```python
from build123d import *

# Parameters (mm, degrees)
BOSS_EXTRUDE1_DEPTH            = 2.54
F_3_16_0_1875_DIAMETER_HOLE1_D = 4.7625
CHAMFER1_SIZE                  = 2.54
CHAMFER2_SIZE                  = 0.2


with BuildPart() as part:
    # Sketch1 → Boss-Extrude1 (new body)
    with BuildSketch(Plane(origin=(0, 0, 0), x_dir=(1, 0, 0), z_dir=(0, 1, 0))):
        Polygon((0, 0), (-25.4, 0), (-25.4, -25.4), (50.8, -25.4), (50.8, 0), (25.4, 0), (25.4, 50.8), (0, 50.8), align=None)
    extrude(amount=BOSS_EXTRUDE1_DEPTH)

    # 3/16 (0.1875) Diameter Hole1 (through all)
    with Locations(Plane(origin=(0, 2.54, 0), x_dir=(1, 0, 0), z_dir=(0, 1, 0))):
        with Locations((12.7, 38.1), (12.7, 12.7), (12.7, -12.7), (38.1, -12.7), (-12.7, -12.7)):
            Hole(F_3_16_0_1875_DIAMETER_HOLE1_D / 2)

    # Chamfer1
    chamfer1_edges = [part.edges().sort_by_distance(p)[0] for p in [
        (0, 1.27, -50.8),
        (25.4, 1.27, -50.8),
        (25.4, 1.27, 0),
        (50.8, 1.27, 0),
        (50.8, 1.27, 25.4),
        (-25.4, 1.27, 25.4),
        (-25.4, 1.27, 0),
        (0, 1.27, 0),
    ]]
    chamfer(chamfer1_edges, length=CHAMFER1_SIZE)

    # Chamfer2
    chamfer2_edges = [part.edges().sort_by_distance(p)[0] for p in [
        (-10.31875, 2.54, 12.7),
        (-10.31875, 0, 12.7),
        (40.48125, 2.54, 12.7),
        (40.48125, 0, 12.7),
        (15.08125, 2.54, 12.7),
        (15.08125, 0, 12.7),
        (15.08125, 2.54, -12.7),
        (15.08125, 0, -12.7),
        (15.08125, 2.54, -38.1),
        (15.08125, 0, -38.1),
    ]]
    chamfer(chamfer2_edges, length=CHAMFER2_SIZE)


solid = part.part
```
Here's how the part is built. I have some questions about the finished solid (model axes, mm). A direction names the side the tool comes from. Coordinates: 2 decimals unless noted, no trailing zeros. Loops run counter-clockwise (first coordinate to the right, second up) from the corner with the lowest first, then second, coordinate; pieces in that order, holes last. Notation, with made-up numbers: (83.25, 88) - (104.25, 88) arc R35 ccw to (104.25, 125) - close; hole circle Ø3 at (-14, 65). An arc over 180 degrees is marked (long way). Return JSON: item names as keys, results as strings. Group by question number.
Item 1: If we section it at D-D on x = 38.1: Write out the boundary of the cut face in (y, z).
Item 2: If we section it at B-B on y = 0.85: Write out the boundary of the cut face in (x, z), and give its area (3 significant figures).
Item 3: On a 3-axis mill with a long thin cutter (end or side, diameter ignored), from which of +Z, -Z, +X, -X, +Y, -Y can I reach the whole of each face in a straight line? I mean faces 5 (the face through (0, 1, -26)), 6 (the face through (38, 1, 0)), 7 (the face through (12, 1, 25.4)). Say none if no direction works.
Item 4: I need wall thicknesses on line 1 (Z direction, x = 12.7, y = 0.75); line 2 (X direction, y = 1.7, z = 12.7); line 3 (Z direction, x = 38.1, y = 1.85). Which ranges of each line are inside material? Lowest first, please. Write a range as from..to.
Item 5: We'd pull the mould along Z, two halves only. Please class faces 1 (the face through (50.8, 1, 13)), 2 (the face through (49.51, 1.25, 1.25)), 3 (the face through (-13.98, 1.26, 10.69)), 4 (the face through (11.42, 1.26, -14.71)): +Z half, -Z half, draft (parallel to the pull), parting line (faces both ways), or undercut.
Item 6: Will these pins go through, and if not, where does the flat tip stop? P1, Ø1, axis at x = 0, y = 0.5, coming from the -Z side; P2, Ø1.3, axis at y = 1, z = -19.5, coming from the +X side.
Item 7: If we section it at C-C on z = -38.1: Write out the boundary of the cut face in (x, y), and give its area (3 significant figures).
Item 8: If we section it at A-A on z = 12.7: Write out the boundary of the cut face in (x, y).
Calculated:
{
 "1": {"outline": "(0, 0) - (2.54, 0) - (2.54, 10.12) - (2.34, 10.32) - (0.2, 10.32) - (0, 10.12) - close; (0, 15.28) - (0.2, 15.08) - (2.34, 15.08) - (2.54, 15.28) - (2.54, 25.4) - (0, 25.4) - close"},
 "2": {"outline": "(-25.4, 2.54) - (-22.86, 0) - (-2.54, 0) - (0, -2.54) - (0, -48.26) - (2.54, -50.8) - (22.86, -50.8) - (25.4, -48.26) - (25.4, -2.54) - (27.94, 0) - (48.26, 0) - (50.8, 2.54) - (50.8, 22.86) - (48.26, 25.4) - (-22.86, 25.4) - (-25.4, 22.86) - close; hole circle Ø4.76 at (-12.7, 12.7); hole circle Ø4.76 at (12.7, -38.1); hole circle Ø4.76 at (12.7, -12.7); hole circle Ø4.76 at (12.7, 12.7); hole circle Ø4.76 at (38.1, 12.7)", "area": "3,120 mm^2"},
 "3": {"face 5": "-Z, -X, +Y, -Y", "face 6": "-Z, +X, +Y, -Y", "face 7": "+Z, +X, -X, +Y, -Y"},
 "4": {"line 1": "z = -50.8..-40.48, -35.72..-15.08, -10.32..10.32, 15.08..25.4", "line 2": "x = -25.4..-15.08, -10.32..10.32, 15.08..35.72, 40.48..50.8", "line 3": "z = 0..10.32, 15.08..25.4"},
 "5": {"face 1": "draft", "face 2": "-Z half", "face 3": "undercut", "face 4": "undercut"},
 "6": {"P1": "stops at z = -48.76", "P2": "stops at x = 25.4"},
 "7": {"outline": "(0, 0) - (10.12, 0) - (10.32, 0.2) - (10.32, 2.34) - (10.12, 2.54) - (0, 2.54) - close; (15.08, 0.2) - (15.28, 0) - (25.4, 0) - (25.4, 2.54) - (15.28, 2.54) - (15.08, 2.34) - close", "area": "52.3 mm^2"},
 "8": {"outline": "(-25.4, 0) - (-15.28, 0) - (-15.08, 0.2) - (-15.08, 2.34) - (-15.28, 2.54) - (-25.4, 2.54) - close; (-10.32, 0.2) - (-10.12, 0) - (10.12, 0) - (10.32, 0.2) - (10.32, 2.34) - (10.12, 2.54) - (-10.12, 2.54) - (-10.32, 2.34) - close; (15.08, 0.2) - (15.28, 0) - (35.52, 0) - (35.72, 0.2) - (35.72, 2.34) - (35.52, 2.54) - (15.28, 2.54) - (15.08, 2.34) - close; (40.48, 0.2) - (40.68, 0) - (50.8, 0) - (50.8, 2.54) - (40.68, 2.54) - (40.48, 2.34) - close"}
}
